The listing builds one solid part. Answer for the finished solid, in the listing's coordinates (mm). Give positions to 0.01 mm unless a question says otherwise; leave off trailing zeros. One line per question, with ' | ' between items.
Autodesk Inventor part; units mm, degrees
ref_plane "YZ Plane" through (0, 0, 0) normal (1, 0, 0) x (0, 1, 0)
ref_plane "XZ Plane" through (0, 0, 0) normal (0, 1, 0) x (-1, 0, 0)
ref_plane "XY Plane" through (0, 0, 0) normal (0, 0, 1) x (1, 0, 0)
sketch "Sketch1" plane through (0, 0, 0) normal (0, 1, 0) x (-1, 0, 0)
  line L0 (5.872, 162.6948) -> (-5.872, 162.6948)
  line L1 (-5.872, 162.6948) -> (-5.872, -162.6948)
  line L2 (-5.872, -162.6948) -> (5.872, -162.6948)
  line L3 (5.872, -162.6948) -> (5.872, 162.6948)
  line L4 (5.872, 162.6948) -> (-5.872, -162.6948) construction
  line L5 (-5.872, 162.6948) -> (5.872, -162.6948) construction
  circle A0 centre (0, 0) radius 1.85
  circle A1 centre (0, 16) radius 1.85
  circle A2 centre (0, 32) radius 1.85
  circle A3 centre (0, 48) radius 1.85
  circle A4 centre (0, 64) radius 1.85
  circle A5 centre (0, 80) radius 1.85
  circle A6 centre (0, 96) radius 1.85
  circle A7 centre (0, 112) radius 1.85
  circle A8 centre (0, 128) radius 1.85
  circle A9 centre (0, 144) radius 1.85
  circle A10 centre (0, -16) radius 1.85
  circle A11 centre (0, 0) radius 1.85
  circle A12 centre (0, 16) radius 1.85
  circle A13 centre (0, 32) radius 1.85
  circle A14 centre (0, 48) radius 1.85
  circle A15 centre (0, 64) radius 1.85
  circle A16 centre (0, 80) radius 1.85
  circle A17 centre (0, 96) radius 1.85
  circle A18 centre (0, 112) radius 1.85
  circle A19 centre (0, 128) radius 1.85
  circle A20 centre (0, -32) radius 1.85
  circle A21 centre (0, -16) radius 1.85
  circle A22 centre (0, 0) radius 1.85
  circle A23 centre (0, 16) radius 1.85
  circle A24 centre (0, 32) radius 1.85
  circle A25 centre (0, 48) radius 1.85
  circle A26 centre (0, 64) radius 1.85
  circle A27 centre (0, 80) radius 1.85
  circle A28 centre (0, 96) radius 1.85
  circle A29 centre (0, 112) radius 1.85
  circle A30 centre (0, -48) radius 1.85
  circle A31 centre (0, -32) radius 1.85
  circle A32 centre (0, -16) radius 1.85
  circle A33 centre (0, 0) radius 1.85
  circle A34 centre (0, 16) radius 1.85
  circle A35 centre (0, 32) radius 1.85
  circle A36 centre (0, 48) radius 1.85
  circle A37 centre (0, 64) radius 1.85
  circle A38 centre (0, 80) radius 1.85
  circle A39 centre (0, 96) radius 1.85
  circle A40 centre (0, -64) radius 1.85
  circle A41 centre (0, -48) radius 1.85
  circle A42 centre (0, -32) radius 1.85
  circle A43 centre (0, -16) radius 1.85
  circle A44 centre (0, 0) radius 1.85
  circle A45 centre (0, 16) radius 1.85
  circle A46 centre (0, 32) radius 1.85
  circle A47 centre (0, 48) radius 1.85
  circle A48 centre (0, 64) radius 1.85
  circle A49 centre (0, 80) radius 1.85
  circle A50 centre (0, -80) radius 1.85
  circle A51 centre (0, -64) radius 1.85
  circle A52 centre (0, -48) radius 1.85
  circle A53 centre (0, -32) radius 1.85
  circle A54 centre (0, -16) radius 1.85
  circle A55 centre (0, 0) radius 1.85
  circle A56 centre (0, 16) radius 1.85
  circle A57 centre (0, 32) radius 1.85
  circle A58 centre (0, 48) radius 1.85
  circle A59 centre (0, 64) radius 1.85
  circle A60 centre (0, -96) radius 1.85
  circle A61 centre (0, -80) radius 1.85
  circle A62 centre (0, -64) radius 1.85
  circle A63 centre (0, -48) radius 1.85
  circle A64 centre (0, -32) radius 1.85
  circle A65 centre (0, -16) radius 1.85
  circle A66 centre (0, 0) radius 1.85
  circle A67 centre (0, 16) radius 1.85
  circle A68 centre (0, 32) radius 1.85
  circle A69 centre (0, 48) radius 1.85
  circle A70 centre (0, -112) radius 1.85
  circle A71 centre (0, -96) radius 1.85
  circle A72 centre (0, -80) radius 1.85
  circle A73 centre (0, -64) radius 1.85
  circle A74 centre (0, -48) radius 1.85
  circle A75 centre (0, -32) radius 1.85
  circle A76 centre (0, -16) radius 1.85
  circle A77 centre (0, 0) radius 1.85
  circle A78 centre (0, 16) radius 1.85
  circle A79 centre (0, 32) radius 1.85
  circle A80 centre (0, -128) radius 1.85
  circle A81 centre (0, -112) radius 1.85
  circle A82 centre (0, -96) radius 1.85
  circle A83 centre (0, -80) radius 1.85
  circle A84 centre (0, -64) radius 1.85
  circle A85 centre (0, -48) radius 1.85
  circle A86 centre (0, -32) radius 1.85
  circle A87 centre (0, -16) radius 1.85
  circle A88 centre (0, 0) radius 1.85
  circle A89 centre (0, 16) radius 1.85
  circle A90 centre (0, -144) radius 1.85
  circle A91 centre (0, -128) radius 1.85
  circle A92 centre (0, -112) radius 1.85
  circle A93 centre (0, -96) radius 1.85
  circle A94 centre (0, -80) radius 1.85
  circle A95 centre (0, -64) radius 1.85
  circle A96 centre (0, -48) radius 1.85
  circle A97 centre (0, -32) radius 1.85
  circle A98 centre (0, -16) radius 1.85
  circle A99 centre (0, 0) radius 1.85
  dimension "d0" = 3.7
  dimension "d3" = 16
  dimension "d6" = 16
extrude "Extrusion1" add sketch "Sketch1" along normal blind 6.35
properties part number "ServoArm"
Item 1: Find section A-A (y = 2.5). Count the separate pieces of the cut face and the enclosed holes in it, then the cut area to 3 significant figures.
Answers below:
separate pieces: 1 | enclosed holes: 19 | area: 3,620 mm²
Item 2: A flat-ended cylindrical pin translates along its axis: pin 1 (3 mm diameter, centred on x = 0, z = -112, fed in from +Y). Find the tip coordinate at first contact, or state that the pin passes through.
Answers below:
pin 1: through
Item 3: Consider line 1 (X direction, y = 3.5, z = -112). Determine where the line is inside the solid, lowest interval first. Write a range as [from, to].
Answers below:
line 1: [-5.87, -1.85], [1.85, 5.87]
